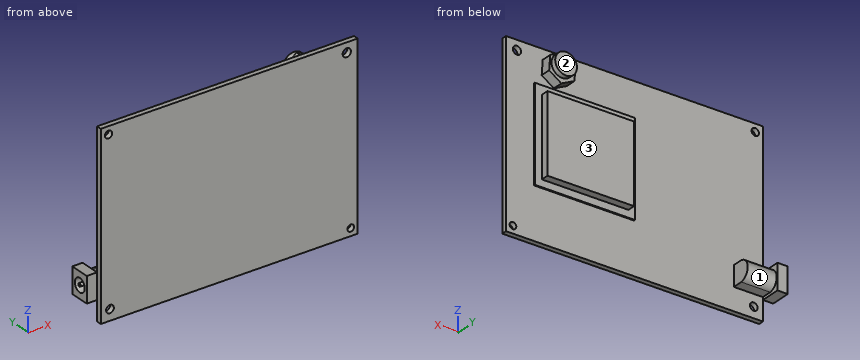
```python
from build123d import *

# Parameters (mm, degrees)
SKETCH1_W            = 100
SKETCH1_H            = 70
BOSS_EXTRUDE2_DEPTH  = 2
SKETCH2_R            = 1.51253395
CUT_EXTRUDE3_DEPTH   = 3
SKETCH3_R            = 1.435290784
CUT_EXTRUDE4_DEPTH   = 3
SKETCH4_R            = 1.301317422
CUT_EXTRUDE5_DEPTH   = 3
SKETCH5_R            = 1.616299526
CUT_EXTRUDE6_DEPTH   = 3
SKETCH6_W            = 17.296093804
SKETCH6_H            = 7.856677749
BOSS_EXTRUDE3_DEPTH  = 7.5
CUT_EXTRUDE14_DEPTH  = 19
CUT_EXTRUDE15_DEPTH  = 19
SKETCH15_W           = 9.915871842
SKETCH15_H           = 7.754440815
BOSS_EXTRUDE6_DEPTH  = 4
SKETCH16_R           = 2.634959219
CUT_EXTRUDE16_DEPTH  = 7
SKETCH17_R           = 0.632651109
BOSS_EXTRUDE7_DEPTH  = 7
SKETCH18_W           = 38.944699871
SKETCH18_H           = 36.600864012
BOSS_EXTRUDE8_DEPTH  = 0.5
SKETCH19_W           = 33.712674361
SKETCH19_H           = 30.360976244
BOSS_EXTRUDE9_DEPTH  = 3
SKETCH20_R           = 4.233704758
BOSS_EXTRUDE10_DEPTH = 6
BOSS_EXTRUDE11_DEPTH = 4


with BuildPart() as part:
    # Sketch1 → Boss-Extrude2 (new body)
    with BuildSketch(Plane(origin=(0, 0, 0), x_dir=(1, 0, 0), z_dir=(0, 1, 0))):
        Rectangle(SKETCH1_W, SKETCH1_H)
    extrude(amount=BOSS_EXTRUDE2_DEPTH)

    # Sketch2 → Cut-Extrude3 (cut)
    with BuildSketch(Plane(origin=(0, 2, 0), x_dir=(1, 0, 0), z_dir=(0, 1, 0))):
        with Locations(Location((-46.439620532, 30.814260712, 0), (0, 0, 270))):
            Circle(SKETCH2_R)
    extrude(amount=-CUT_EXTRUDE3_DEPTH, mode=Mode.SUBTRACT)

    # Sketch3 → Cut-Extrude4 (cut)
    with BuildSketch(Plane(origin=(0, 2, 0), x_dir=(1, 0, 0), z_dir=(0, 1, 0))):
        with Locations(Location((-47.004076073, -32.008947101, 0), (0, 0, 270))):
            Circle(SKETCH3_R)
    extrude(amount=-CUT_EXTRUDE4_DEPTH, mode=Mode.SUBTRACT)

    # Sketch4 → Cut-Extrude5 (cut)
    with BuildSketch(Plane(origin=(0, 2, 0), x_dir=(1, 0, 0), z_dir=(0, 1, 0))):
        with Locations(Location((47.302855544, 32.117059369, 0), (0, 0, 270))):
            Circle(SKETCH4_R)
    extrude(amount=-CUT_EXTRUDE5_DEPTH, mode=Mode.SUBTRACT)

    # Sketch5 → Cut-Extrude6 (cut)
    with BuildSketch(Plane(origin=(0, 2, 0), x_dir=(1, 0, 0), z_dir=(0, 1, 0))):
        with Locations(Location((45.747085663, -31.267682523, 0), (0, 0, 270))):
            Circle(SKETCH5_R)
    extrude(amount=-CUT_EXTRUDE6_DEPTH, mode=Mode.SUBTRACT)

    # Sketch6 → Boss-Extrude3 (add)
    with BuildSketch(Plane(origin=(0, 2, 0), x_dir=(1, 0, 0), z_dir=(0, 1, 0))):
        with Locations((-47.333268099, 22.322741547)):
            Rectangle(SKETCH6_W, SKETCH6_H)
    extrude(amount=BOSS_EXTRUDE3_DEPTH)

    # Sketch13 → Cut-Extrude14 (cut)
    with BuildSketch(Plane.ZY.offset(55.981315001)):
        with BuildLine():
            Line((-18.394402672, 9.5), (-26.251080421, 9.5))
            Line((-26.251080421, 9.5), (-26.251080421, 5.951221756))
            ThreePointArc((-26.251080421, 5.951221756), (-22.211334605, 9.370260294), (-18.394402672, 5.704144993))
            Line((-18.394402672, 5.704144993), (-18.394402672, 9.5))
        make_face()
    extrude(amount=-CUT_EXTRUDE14_DEPTH, mode=Mode.SUBTRACT)

    # Sketch14 → Cut-Extrude15 (cut)
    with BuildSketch(Plane(origin=(0, 2, 0), x_dir=(-1, 0, 0), z_dir=(0, -1, 0))):
        Polygon((49.983450697, 17.629135674), (49.983450697, 26.82990783), (57.169456537, 26.82990783), (57.911353863, 13.473102082), align=None)
    extrude(amount=-CUT_EXTRUDE15_DEPTH, mode=Mode.SUBTRACT)

    # Sketch15 → Boss-Extrude6 (add)
    with BuildSketch(Plane.ZY.offset(49.983450697)):
        with Locations((-22.336364996, 5.892577674)):
            Rectangle(SKETCH15_W, SKETCH15_H)
    extrude(amount=BOSS_EXTRUDE6_DEPTH)

    # Sketch16 → Cut-Extrude16 (cut)
    with BuildSketch(Plane.ZY.offset(53.983450697)):
        with Locations((-22.358887933, 5.764755063)):
            Circle(SKETCH16_R)
    extrude(amount=-CUT_EXTRUDE16_DEPTH, mode=Mode.SUBTRACT)

    # Sketch17 → Boss-Extrude7 (add)
    with BuildSketch(Plane.ZY.offset(46.983450697)):
        with Locations((-22.320088974, 5.946166612)):
            Circle(SKETCH17_R)
    extrude(amount=BOSS_EXTRUDE7_DEPTH)

    # Sketch18 → Boss-Extrude8 (add)
    with BuildSketch(Plane(origin=(0, 2, 0), x_dir=(1, 0, 0), z_dir=(0, 1, 0))):
        with Locations((19.693389893, -3.245226769)):
            Rectangle(SKETCH18_W, SKETCH18_H)
    extrude(amount=BOSS_EXTRUDE8_DEPTH)

    # Sketch19 → Boss-Extrude9 (add)
    with BuildSketch(Plane(origin=(0, 2.5, 0), x_dir=(1, 0, 0), z_dir=(0, 1, 0))):
        with Locations((19.582517613, -2.921097191)):
            Rectangle(SKETCH19_W, SKETCH19_H)
    extrude(amount=BOSS_EXTRUDE9_DEPTH)

    # Sketch20 → Boss-Extrude10 (add)
    with BuildSketch(Plane(origin=(0, 2, 0), x_dir=(1, 0, 0), z_dir=(0, 1, 0))):
        with Locations(Location((30.998863529, -28.543635421, 0), (0, 0, 270))):
            Circle(SKETCH20_R)
    extrude(amount=BOSS_EXTRUDE10_DEPTH)

    # Sketch21 → Boss-Extrude11 (add)
    with BuildSketch(Plane(origin=(0, 2, 0), x_dir=(1, 0, 0), z_dir=(0, 1, 0))):
        Polygon((35.70636757, -31.11116693), (36.11182012, -25.437321781), (31.400852359, -22.249266998), (26.284432048, -24.735057364), (25.878979498, -30.408902513), (30.589947259, -33.596957296), align=None)
    extrude(amount=BOSS_EXTRUDE11_DEPTH)


solid = part.part
```
CAD build for the part. Positions are in the model's coordinates, mm. Face numbers are marked on the shaded views. A direction names the side the tool comes from. Coordinates: 2 decimals unless noted, no trailing zeros. Write each loop counter-clockwise with the first axis right and the second up, starting at its lowest first coordinate (ties: lowest second). Pieces come first, ordered by that corner, then holes.
(1) Cut at B-B, the plane x = 11. List the corners of the cut face in (y, z).
(2) Drill centre lines: probe 1 along X at (y, z) = (4.5, -18); probe 2 along Z at (x, y) = (5, 3.75); probe 3 along Y at (x, z) = (-23.5, 6). Where is each one in solid material? Low to high.
(3) 3-axis set-ups, long thin cutter, end or side, ignore diameter. For the marked faces 1, 2 and 3: which of +Z, -Z, +X, -X, +Y, -Y reach the whole face in a straight line?
(4) Cut at C-C, the plane z = -5. List the corners of the cut face in (x, y), and give its area (3 significant figures).
(5) Cut at D-D, the plane x = -37.5. List the corners of the cut face in (y, z), and give its area (3 significant figures).
(6) Flat gauge pins, fed straight in: pin 1 (4 mm diameter, centred on x = -14.5, z = -23.5, fed in from +Y); pin 2 (15 mm diameter, centred on x = 27, z = -4.5, fed in from +Y); pin 3 (11.5 mm diameter, centred on x = 29, z = 26.5, fed in from +Y); pin 4 (2.5 mm diameter, centred on x = -46.44, z = -30.81, fed in from +Y). Where does each tip first touch, or does it go through?
(7) Cut at A-A, the plane y = 4.25. List the corners of the cut face in (x, z), and give its area (3 significant figures).
Geometry says:
1. outline: (0, -35) - (2, -35) - (2, -15.06) - (2.5, -15.06) - (2.5, -12.26) - (5.5, -12.26) - (5.5, 18.1) - (2.5, 18.1) - (2.5, 21.55) - (2, 21.55) - (2, 35) - (0, 35) - close
2. probe 1: x = -53.98 to -49.98
2. probe 2: z = -12.26 to 18.1
2. probe 3: y = 0 to 2
3. face 1: +X, +Y
3. face 2: +Z, -Z, +X, -X, +Y
3. face 3: -Z, +X, -X, +Y
4. outline: (-50, 0) - (50, 0) - (50, 2) - (39.17, 2) - (39.17, 2.5) - (36.44, 2.5) - (36.44, 5.5) - (2.73, 5.5) - (2.73, 2.5) - (0.22, 2.5) - (0.22, 2) - (-50, 2) - close
4. area: 321 mm2
5. outline: (0, -35) - (2, -35) - (2, 35) - (0, 35) - close
5. area: 140 mm2
6. pin 1: stops at y = 2
6. pin 2: stops at y = 5.5
6. pin 3: stops at y = 8
6. pin 4: passes through
7. outline: (-53.98, -27.29) - (-49.98, -27.29) - (-49.98, -26.25) - (-38.69, -26.25) - (-38.69, -18.39) - (-49.98, -18.39) - (-49.98, -17.38) - (-53.98, -17.38) - (-53.98, -20.2) - (-46.98, -20.2) - (-46.98, -24.51) - (-53.98, -24.51) - close; (2.73, -12.26) - (36.44, -12.26) - (36.44, 18.1) - (2.73, 18.1) - close; (25.88, 30.41) - (26.28, 24.74) - (31.4, 22.25) - (36.11, 25.44) - (35.71, 31.11) - (30.59, 33.6) - close
7. area: 1,210 mm2
